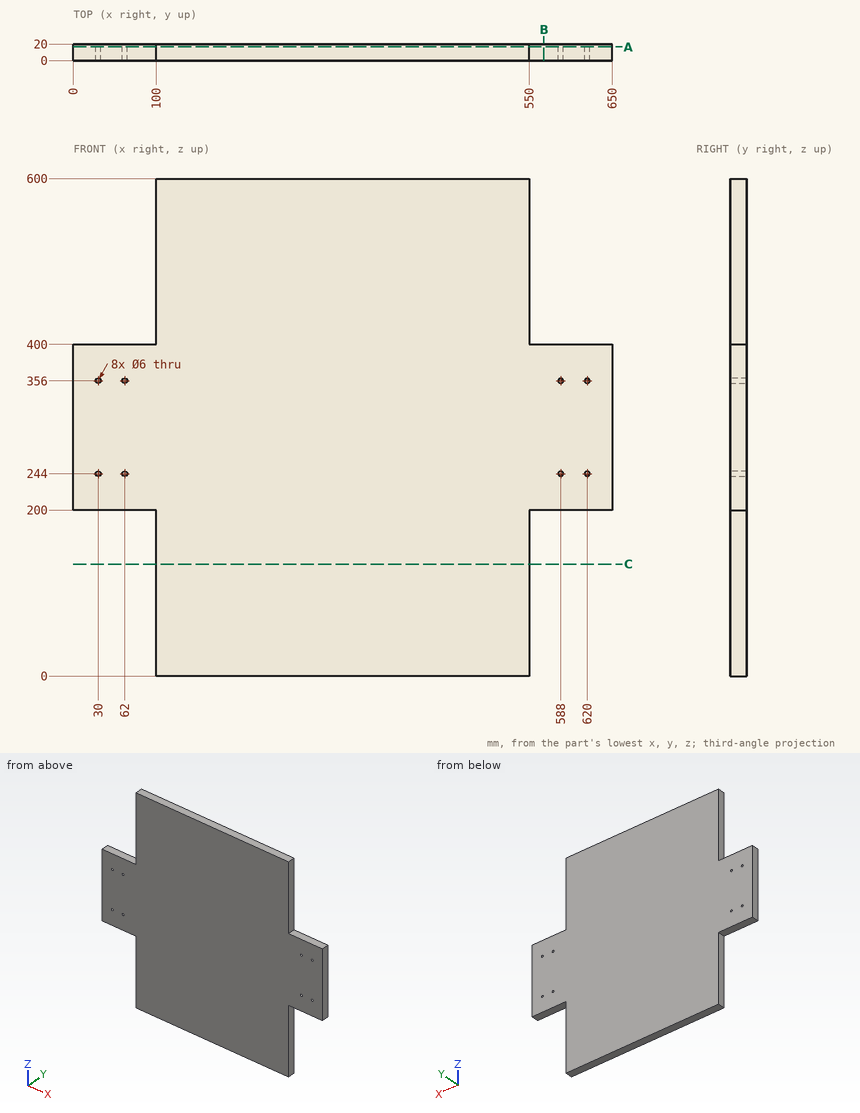
Here's the drawing with two shaded views (mm, measured from the low corner). I have some questions. Coordinates: 2 decimals unless noted, no trailing zeros. Order: outer loops, then holes, each group sorted by start corner. A loop starts at its lowest first (then second) coordinate and runs counter-clockwise, first axis right, second up. Notation, with made-up numbers: (-2.5, 87) - (9.5, 87) arc R17 cw to (9.5, 119) - close; hole circle Ø5 at (14.25, 81). An arc over 180 degrees is marked (long way). Answer in a Markdown table with one row per item.
1. If I drill on line 1 along Z through (x, y) = (62, 11.5); line 2 along X through (y, z) = (12.75, 244); line 3 along X through (y, z) = (19, 49), over which ranges is the centre line in solid material (lowest first)?
Reply:
| item | result |
|---|---|
| line 1 | z = 200 to 241, 247 to 353, 359 to 400 |
| line 2 | x = 0 to 27, 33 to 59, 65 to 585, 591 to 617, 623 to 650 |
| line 3 | x = 100 to 550 |
2. For pin 1 (1.5 mm diameter, centred on y = 6, z = 136.5, fed in from +X); pin 2 (10 mm diameter, centred on x = 64.5, y = 12.5, fed in from +Z); pin 3 (5 mm diameter, centred on y = 4.5, z = 403.5, fed in from -X), each with a flat end and sliding along its axis, tell me the tip position at first contact or that it passes through.
Reply:
| item | result |
|---|---|
| pin 1 | stops at x = 550 |
| pin 2 | stops at z = 400 |
| pin 3 | stops at x = 100 |
3. Suppose I cut it at C-C (z = 135). Please give me the cut outline in (x, y), and give its area (3 significant figures).
Reply:
| item | result |
|---|---|
| outline | (100, 0) - (550, 0) - (550, 20) - (100, 20) - close |
| area | 9,000 mm^2 |
4. Suppose I cut it at A-A (y = 16.5). Give the number of separate pieces and of enclosed holes in the cut face, and give its area (3 significant figures).
Reply:
| item | result |
|---|---|
| separate pieces | 1 |
| enclosed holes | 8 |
| area | 310,000 mm^2 |
5. Suppose I cut it at B-B (x = 567.5). Please give me the cut outline in (y, z).
Reply:
| item | result |
|---|---|
| outline | (0, 200) - (20, 200) - (20, 400) - (0, 400) - close |
